The listing builds one solid part. Answer for the finished solid, in the listing's coordinates (mm). Give positions to 0.01 mm unless a question says otherwise; leave off trailing zeros. Order: outer loops, then holes, each group sorted by start corner. A loop starts at its lowest first (then second) coordinate and runs counter-clockwise, first axis right, second up. Notation, with made-up numbers: (-40, -9) -> (15, -9) arc R25 ccw to (15, 24) -> close; hole circle Ø8 at (82, 33). An arc over 180 degrees is marked (long way). One line per question, with ' | ' between items. Start each with the question number.
```python
from build123d import *

# Parameters (mm, degrees)
CROQUIS1_R              = 2.55
CROQUIS1_R_2            = 1.55
SALIENTE_EXTRUIR1_DEPTH = 3
REDONDEO2_R             = 2
CORTAR_EXTRUIR1_DEPTH   = 3


with BuildPart() as part:
    # Croquis1 → Saliente-Extruir1 (new body)
    with BuildSketch(Plane(origin=(0, 0, 0), x_dir=(1, 0, 0), z_dir=(0, 1, 0))):
        Polygon((0, 0), (200, 0), (200, 30), (192, 30), (192, 38), (178, 38), (178, 30), (115, 30), (115, 35), (85, 35), (85, 30), (22, 30), (22, 38), (8, 38), (8, 30), (0, 30), align=None)
        with Locations((3.4, 26.6)):
            Circle(CROQUIS1_R, mode=Mode.SUBTRACT)
        with Locations((26.6, 26.6)):
            Circle(CROQUIS1_R, mode=Mode.SUBTRACT)
        with Locations((26.6, 3.4)):
            Circle(CROQUIS1_R, mode=Mode.SUBTRACT)
        with Locations((3.4, 3.4)):
            Circle(CROQUIS1_R, mode=Mode.SUBTRACT)
        with Locations((173.4, 3.4)):
            Circle(CROQUIS1_R, mode=Mode.SUBTRACT)
        with Locations((196.6, 3.4)):
            Circle(CROQUIS1_R, mode=Mode.SUBTRACT)
        with Locations((196.6, 26.6)):
            Circle(CROQUIS1_R, mode=Mode.SUBTRACT)
        with Locations((173.4, 26.6)):
            Circle(CROQUIS1_R, mode=Mode.SUBTRACT)
        with Locations((100, 30)):
            Circle(CROQUIS1_R_2, mode=Mode.SUBTRACT)
        with Locations((100, 10)):
            Circle(CROQUIS1_R_2, mode=Mode.SUBTRACT)
        with Locations((70, 23)):
            Circle(CROQUIS1_R_2, mode=Mode.SUBTRACT)
        with Locations((70, 8)):
            Circle(CROQUIS1_R_2, mode=Mode.SUBTRACT)
        with Locations((130, 8)):
            Circle(CROQUIS1_R_2, mode=Mode.SUBTRACT)
        with Locations((130, 23)):
            Circle(CROQUIS1_R_2, mode=Mode.SUBTRACT)
    extrude(amount=SALIENTE_EXTRUIR1_DEPTH)

    # Redondeo2
    redondeo2_edges = [part.edges().sort_by_distance(p)[0] for p in [
        (0, 1.5, -30),
        (8, 1.5, -30),
        (8, 1.5, -38),
        (22, 1.5, -38),
        (22, 1.5, -30),
        (85, 1.5, -30),
        (85, 1.5, -35),
        (115, 1.5, -35),
        (115, 1.5, -30),
        (178, 1.5, -30),
        (178, 1.5, -38),
        (192, 1.5, -38),
        (192, 1.5, -30),
        (200, 1.5, -30),
        (200, 1.5, 0),
        (0, 1.5, 0),
    ]]
    fillet(redondeo2_edges, radius=REDONDEO2_R)

    # Croquis2 → Cortar-Extruir1 (cut)
    with BuildSketch(Plane(origin=(0, 3, 0), x_dir=(1, 0, 0), z_dir=(0, 1, 0))):
        with BuildLine():
            Line((85, 0), (115, 0))
            Line((115, 0), (115, 1.5))
            ThreePointArc((115, 1.5), (114.707106781, 2.207106781), (114, 2.5))
            Line((114, 2.5), (86, 2.5))
            ThreePointArc((86, 2.5), (85.292893219, 2.207106781), (85, 1.5))
            Line((85, 1.5), (85, 0))
        make_face()
    extrude(amount=-CORTAR_EXTRUIR1_DEPTH, mode=Mode.SUBTRACT)


solid = part.part
```
(1) Consider line 1 (Z direction, x = 70, y = 1.5); line 2 (X direction, y = 1.9, z = -32); line 3 (X direction, y = 2.35, z = -8). Determine where each line is inside the solid, lowest interval first.
(2) Given P1, Ø3, axis at x = 196.6, z = -26.6, coming from the +Y side; P2, Ø0.8, axis at y = 2, z = -32.5, coming from the -X side; P3, Ø1.5, axis at x = 57.5, y = 2, coming from the -Z side; P4, Ø0.8, axis at y = 2, z = -32.5, coming from the +X side, each flat-ended and moving along its own axis, determine where each tip first touches the part or whether it passes through.
(3) Determine the mould class of faces 1 (the face through (194.052, 1.479, -3.512)), 2 (the face through (29.03, 1.48, -4.17)), 3 (the face through (99, 3, -15)) for opening direction Z: pulls with the +Z half, pulls with the -Z half, needs draft (parallel to the pull), parting line crosses it, or undercut.
(4) The part is cut by section A-A on y = 0.55. State how many separate pieces and enclosed holes the cut face has, plus the area to 3 significant figures.
(5) The part is cut by section B-B on x = 145.5. Determine the outline of the cut face in (y, z).
Result sheet:
1) line 1: z = -30 to -24.55, -21.45 to -9.55, -6.45 to 0 | line 2: x = 8 to 22, 85 to 115, 178 to 192 | line 3: x = 0 to 68.45, 71.55 to 128.45, 131.55 to 200
2) P1: passes through | P2: stops at x = 8 | P3: stops at z = -30 | P4: stops at x = 192
3) face 1: undercut | face 2: undercut | face 3: needs draft
4) separate pieces: 1 | enclosed holes: 14 | area: 6,090 mm^2
5) outline: (0, -30) -> (3, -30) -> (3, 0) -> (0, 0) -> close
